Part model, mm, in its own coordinate system. Face numbers are marked on the shaded views. A direction names the side the tool comes from. Round coordinates to 2 decimals unless told otherwise and drop trailing zeros. Write each loop counter-clockwise with the first axis right and the second up, starting at its lowest first coordinate (ties: lowest second). Pieces come first, ordered by that corner, then holes. Notation, with made-up numbers: (71.25, -20) -> (82.25, -20) arc R9 ccw to (82.25, -6) -> close; hole circle Ø10 at (37.25, 32.25). An arc over 180 degrees is marked (long way). Return JSON: item names as keys, results as strings. Group by question number.
(1) Saw through at A-A (y = 0). List the corners of the cut face in (x, z), plus the area to 3 significant figures.
(2) Tool access for the marked faces 1 and 2: list every direction of +Z, -Z, +X, -X, +Y, -Y with a clear straight run to the whole face (end or side of a thin tool).
(3) Saw through at D-D (x = -29). List the corners of the cut face in (y, z), plus the area to 3 significant figures.
(4) Saw through at C-C (x = -150). List the corners of the cut face in (y, z).
(5) Drop flat-ended pins along their axis: pin 1 Ø2 at (x, z) = (-128, 6.5) entering from +Y; pin 2 Ø1.5 at (x, z) = (-65.5, 5.5) entering from +Y; pin 3 Ø4 at (x, z) = (-29, 34.5) entering from +Y. Give the stop position or say it passes through.
(6) Drill centre lines: L1, parallel to X at y = -34, z = 6; L2, parallel to X at y = 15, z = -25; L3, parallel to X at y = 16, z = -38. Where is each one in solid material? Low to high. Write a range as from..to.
from build123d import *


with BuildPart() as part:
    # Sketch1 → Revolve1 (revolve)
    with BuildSketch(Plane(origin=(0, 0, 0), x_dir=(-1, 0, 0), z_dir=(0, 1, 0))):
        with BuildLine():
            Line((0, 0), (0, 45))
            Line((0, 45), (5, 45))
            Line((5, 45), (5, 39))
            Line((5, 39), (51, 39))
            Line((51, 39), (51, 38))
            Line((51, 38), (61, 38))
            Line((61, 38), (61, 36))
            ThreePointArc((61, 36), (72, 25), (83, 36))
            Line((83, 36), (131, 36))
            Line((131, 36), (131, 32.5))
            Line((131, 32.5), (163, 32.5))
            Line((163, 32.5), (163, 0))
            Line((163, 0), (0, 0))
        make_face()
    revolve(axis=Axis((-163, 0, 0), (1, 0, 0)))


solid = part.part
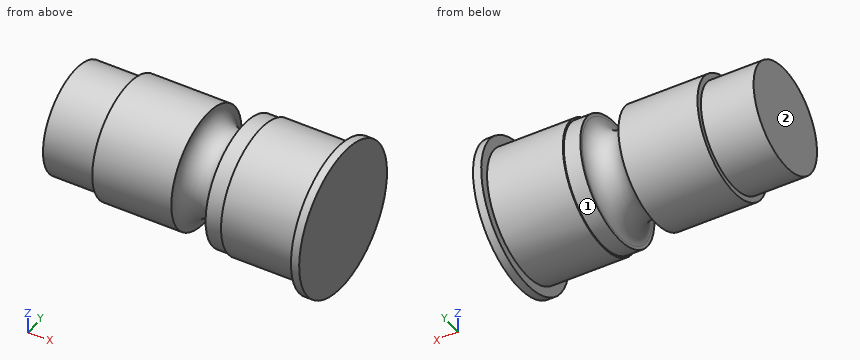
Computed values:
{
 "1": {"outline": "(-163, -32.5) -> (-131, -32.5) -> (-131, -36) -> (-83, -36) arc R11 cw to (-61, -36) -> (-61, -38) -> (-51, -38) -> (-51, -39) -> (-5, -39) -> (-5, -45) -> (0, -45) -> (0, 45) -> (-5, 45) -> (-5, 39) -> (-51, 39) -> (-51, 38) -> (-61, 38) -> (-61, 36) arc R11 cw to (-83, 36) -> (-131, 36) -> (-131, 32.5) -> (-163, 32.5) -> close", "area": "11,500 mm2"},
 "2": {"face 1": "-X", "face 2": "+Z, -Z, -X, +Y, -Y"},
 "3": {"outline": "circle Ø78 at (0, 0)", "area": "4,780 mm2"},
 "4": {"outline": "circle Ø65 at (0, 0)"},
 "5": {"pin 1": "y = 35.58", "pin 2": "y = 27.19", "pin 3": "y = 21.56"},
 "6": {"L1": "-131..-82.9, -61.1..0", "L2": "-163..-80.61, -63.39..0", "L3": "-5..0"}
}
